from build123d import *

# Parameters (mm, degrees)
SKETCH_W     = 60
SKETCH_H     = 60
SKETCH_R     = 1.5
PAD_DEPTH    = 3
SKETCH001_W  = 3
SKETCH001_H  = 22.5
PAD001_DEPTH = 32.5
SKETCH002_R  = 1.1
POCKET_DEPTH = 60


with BuildPart() as part:
    # Sketch → Pad (new body)
    with BuildSketch(Plane.XY):
        Rectangle(SKETCH_W, SKETCH_H)
        with Locations((0, 17.5)):
            Circle(SKETCH_R, mode=Mode.SUBTRACT)
        with Locations((0, 5)):
            Circle(SKETCH_R, mode=Mode.SUBTRACT)
        with Locations((0, -7.5)):
            Circle(SKETCH_R, mode=Mode.SUBTRACT)
        with Locations((0, -20)):
            Circle(SKETCH_R, mode=Mode.SUBTRACT)
        with Locations((-6.25, 11.25)):
            Circle(SKETCH_R, mode=Mode.SUBTRACT)
        with Locations((-18.6, 11.25)):
            Circle(SKETCH_R, mode=Mode.SUBTRACT)
        with Locations((6.25, 11.25)):
            Circle(SKETCH_R, mode=Mode.SUBTRACT)
        with Locations((18.6, 11.25)):
            Circle(SKETCH_R, mode=Mode.SUBTRACT)
        with Locations((-18.6, -1.25)):
            Circle(SKETCH_R, mode=Mode.SUBTRACT)
        with Locations((-18.6, -13.75)):
            Circle(SKETCH_R, mode=Mode.SUBTRACT)
        with Locations((18.7, -1.25)):
            Circle(SKETCH_R, mode=Mode.SUBTRACT)
        with Locations((18.6, -13.75)):
            Circle(SKETCH_R, mode=Mode.SUBTRACT)
        with Locations((-6.25, -13.75)):
            Circle(SKETCH_R, mode=Mode.SUBTRACT)
        with Locations((6.25, -13.75)):
            Circle(SKETCH_R, mode=Mode.SUBTRACT)
        with Locations((-6.25, -1.25)):
            Circle(SKETCH_R, mode=Mode.SUBTRACT)
        with Locations((6.35, -1.25)):
            Circle(SKETCH_R, mode=Mode.SUBTRACT)
    extrude(amount=PAD_DEPTH)

    # Sketch001 (on Face21 of Pad) → Pad001 (join)
    with BuildSketch(Plane(origin=(0, 0, 0), x_dir=(1, 0, 0), z_dir=(0, 0, -1))):
        with Locations((-14.7, 10.75)):
            Rectangle(SKETCH001_W, SKETCH001_H)
        with Locations((13, 10.75)):
            Rectangle(SKETCH001_W, SKETCH001_H)
    extrude(amount=PAD001_DEPTH)

    # Sketch002 (on Face18 of Pad001) → Pocket (cut)
    with BuildSketch(Plane.YZ.offset(14.5)):
        with Locations((-18, -23.5)):
            Circle(SKETCH002_R)
        with Locations((-6, -27.5)):
            Circle(SKETCH002_R)
        with Locations((-18, -7.5)):
            Circle(SKETCH002_R)
        with Locations((-14, -27.5)):
            Circle(SKETCH002_R)
    extrude(amount=-POCKET_DEPTH, mode=Mode.SUBTRACT)


solid = part.part
For this review, take the finished solid that the model builds, in its own axes (mm). A direction names the side the tool comes from. Give positions to 0.01 mm unless a question says otherwise; leave off trailing zeros. Loops run counter-clockwise (first coordinate to the right, second up) from the corner with the lowest first, then second, coordinate; pieces in that order, holes last. Notation, with made-up numbers: M 44,-33 L 64,-33 A36 ccw 64,1 Z; hole C -40,-12.5 d10. An arc over 180 degrees is marked long. Put each result on its own line as item: value. Start each with the question number.
(1) Add section B-B, the plane z = -23.5. Write out the cut boundary in (x, y), then the cut area to 3 significant figures.
(2) For pin 1 (3.5 mm diameter, centred on x = -18.6, y = 11.25, fed in from -Z); pin 2 (1.5 mm diameter, centred on x = -14.5, z = -14, fed in from -Y); pin 3 (5 mm diameter, centred on y = -21.5, z = -15.5, fed in from -X), all flat-tipped, find the tip position at first contact; note any pin that passes through.
(3) Add section C-C, the plane x = 19. Write out the cut boundary in (y, z).
(4) The part is to be moulded in two halves that separate along Z. For faces 1 (the cylindrical face through (-14.679, -6.238, -28.574)), 2 (the flat face through (13, -11, -32.5)), 3 (the cylindrical face through (13.02, -18.87, -24.17)), 4 (the cylindrical face through (-7.44, -2.16, 1.48)), say which applies: +Z half, -Z half, draft (parallel to the pull), parting line (faces both ways), or undercut.
(5) Add section D-D, the plane z = -18. Write out the cut boundary in (x, y).
(6) Add section A-A, the plane y = -20. Write out the cut boundary in (x, z).
(7) Machinability: for faces 5 (the flat face through (11.5, -11, -16)), 6 (the flat face through (14.5, -11, -16)), 7 (the flat face through (-16.2, -11, -16)), which of the approach directions +Z, -Z, +X, -X, +Y, -Y give a long, thin tool a straight path to every point of the face, cutting with its end or side? Answer none if there is none.
(8) Wall thickness on L1, parallel to Z at x = 12, y = -18; L2, parallel to X at y = -1.5, z = -25; L3, parallel to Y at x = 18, z = 2: over which ranges is each line inside the solid? List them lowest first.
Result:
1. outline: M -16.2,-22 L -13.2,-22 L -13.2,-19.1 L -16.2,-19.1 Z; M -16.2,-16.9 L -13.2,-16.9 L -13.2,0.5 L -16.2,0.5 Z; M 11.5,-22 L 14.5,-22 L 14.5,-19.1 L 11.5,-19.1 Z; M 11.5,-16.9 L 14.5,-16.9 L 14.5,0.5 L 11.5,0.5 Z
1. area: 122 mm^2
2. pin 1: stops at z = 0
2. pin 2: stops at y = -22
2. pin 3: stops at x = -16.2
3. outline: M -30,0 L -15.2,0 L -15.2,3 L -30,3 Z; M -12.3,0 L -2.72,0 L -2.72,3 L -12.3,3 Z; M 0.22,0 L 9.8,0 L 9.8,3 L 0.22,3 Z; M 12.7,0 L 30,0 L 30,3 L 12.7,3 Z
4. face 1: undercut
4. face 2: -Z half
4. face 3: undercut
4. face 4: draft
5. outline: M -16.2,-22 L -13.2,-22 L -13.2,0.5 L -16.2,0.5 Z; M 11.5,-22 L 14.5,-22 L 14.5,0.5 L 11.5,0.5 Z
6. outline: M -30,0 L -16.2,0 L -16.2,-32.5 L -13.2,-32.5 L -13.2,0 L -1.5,0 L -1.5,3 L -30,3 Z; M 1.5,0 L 11.5,0 L 11.5,-32.5 L 14.5,-32.5 L 14.5,0 L 30,0 L 30,3 L 1.5,3 Z
7. face 5: -Z, +Y, -Y
7. face 6: -Z, +X, +Y, -Y
7. face 7: -Z, -X, +Y, -Y
8. L1: z = -32.5 to -24.6, -22.4 to -8.6, -6.4 to 3
8. L2: x = -16.2 to -13.2, 11.5 to 14.5
8. L3: y = -30 to -15.12, -12.38 to -2.58, 0.08 to 9.88, 12.62 to 30
